Work out the finished part from the listing and answer in its coordinate system (mm). A direction names the side the tool comes from. Coordinates: 2 decimals unless noted, no trailing zeros. Write each loop counter-clockwise with the first axis right and the second up, starting at its lowest first coordinate (ties: lowest second). Pieces come first, ordered by that corner, then holes. Notation, with made-up numbers: (-15.5, 39) -> (34.5, 39) arc R24 cw to (34.5, 68) -> close; hole circle Ø10 at (34.5, -16.5). An arc over 180 degrees is marked (long way). Write each question's results on one line, items separated by ' | '. Start each with the question number.
from build123d import *

# Parameters (mm, degrees)
SKETCH1_R           = 10
BOSS_EXTRUDE1_DEPTH = 3
SKETCH2_R           = 2.5
BOSS_EXTRUDE2_DEPTH = 8
FILLET2_R           = 0.4
SKETCH3_R           = 4.5
SKETCH3_R_2         = 2.5
BOSS_EXTRUDE3_DEPTH = 1
FILLET3_R           = 0.8
FILLET4_R           = 0.8


with BuildPart() as part:
    # Sketch1 → Boss-Extrude1 (new body)
    with BuildSketch(Plane(origin=(0, 0, 0), x_dir=(1, 0, 0), z_dir=(0, 1, 0))):
        with Locations(Location((0, 0, 0), (0, 0, 270))):
            Circle(SKETCH1_R)
    extrude(amount=BOSS_EXTRUDE1_DEPTH)

    # Sketch2 → Boss-Extrude2 (add)
    with BuildSketch(Plane(origin=(0, 3, 0), x_dir=(1, 0, 0), z_dir=(0, 1, 0))):
        with Locations(Location((0, 0, 0), (0, 0, 270))):
            Circle(SKETCH2_R)
    extrude(amount=BOSS_EXTRUDE2_DEPTH)

    # Fillet2
    fillet2_edges = [part.edges().sort_by_distance(p)[0] for p in [
        (0, 0, -10),
        (0, 3, -10),
    ]]
    fillet(fillet2_edges, radius=FILLET2_R)

    # Sketch3 → Boss-Extrude3 (add)
    with BuildSketch(Plane(origin=(0, 3, 0), x_dir=(1, 0, 0), z_dir=(0, 1, 0))):
        with Locations(Location((0, 0, 0), (0, 0, 270))):
            Circle(SKETCH3_R)
        with Locations(Location((0, 0, 0), (0, 0, 270))):
            Circle(SKETCH3_R_2, mode=Mode.SUBTRACT)
    extrude(amount=BOSS_EXTRUDE3_DEPTH)

    # Fillet3
    fillet3_edges = [part.edges().sort_by_distance(p)[0] for p in [
        (0, 3, -4.5),
    ]]
    fillet(fillet3_edges, radius=FILLET3_R)

    # Fillet4
    fillet4_edges = [part.edges().sort_by_distance(p)[0] for p in [
        (0, 4, -4.5),
    ]]
    fillet(fillet4_edges, radius=FILLET4_R)


solid = part.part
1. Find section A-A on y = 1. Give the vertices of the cut face in (x, z), and give its area (3 significant figures).
2. Find section B-B on y = 10.5. Give the vertices of the cut face in (x, z).
3. For faces 1 (the face through (-4, 3, 4)), 2 (the face through (-9.76, 1.48, -2.17)), determine the directions among +Z, -Z, +X, -X, +Y, -Y from which every point of the face is accessible in a straight line to the end or side of a thin tool.
4. Given pin 1 Ø3 at (y, z) = (2.5, 7.5) entering from +X; pin 2 Ø4 at (x, y) = (5.5, 7) entering from +Z; pin 3 Ø5 at (x, y) = (-6.5, 3.5) entering from +Z; pin 4 Ø5 at (x, z) = (4.5, 3.5) entering from +Y, each flat-ended and moving along its own axis, determine where each tip first touches the part or whether it passes through.
5. Find the intervals of material crossed by L1, parallel to Y at x = 7.25, z = -3.25; L2, parallel to X at y = 2.5, z = -8; L3, parallel to X at y = 4.5, z = -2.25, in increasing order.
Ans:
1) outline: circle Ø20 at (0, 0) | area: 314 mm²
2) outline: circle Ø5 at (0, 0)
3) face 1: +Y | face 2: +Y, -Y
4) pin 1: stops at x = 8 | pin 2: passes through | pin 3: stops at z = 9.1 | pin 4: stops at y = 4
5) L1: y = 0 to 3 | L2: x = -6 to 6 | L3: x = -1.09 to 1.09
